Build history of the part. All positions in model axes, mm. Face numbers are marked on the shaded views. A direction names the side the tool comes from. Coordinates: 2 decimals unless noted, no trailing zeros. Order: outer loops, then holes, each group sorted by start corner. A loop starts at its lowest first (then second) coordinate and runs counter-clockwise, first axis right, second up. Notation, with made-up numbers: M -12,78.25 L 14,78.25 A18 ccw 14,102.25 Z; hole C 43,69 d4. An arc over 180 degrees is marked long. Write item = value, one per line. Start each with the question number.
Q1. Band-saw the part on A-A on x = 14.75. Write the cut outline in (y, z), plus the area to 3 significant figures.
Q2. Pull direction X, two halves, no side cores. Call the marked faces 1, 2 and 3: released by +X, released by -X, zero draft, split by the parting line, or undercut.
Q3. 3-axis set-ups, long thin cutter, end or side, ignore diameter. For the marked faces 4 and 5: which of +Z, -Z, +X, -X, +Y, -Y reach the whole face in a straight line?
Q4. Band-saw the part on D-D on y = -5.5. Write the cut outline in (x, z).
Q5. Band-saw the part on C-C on y = -7.5. Write the cut outline in (x, z).
Q6. Pin check, flat tips, straight feed: P1, Ø7, axis at x = 12.5, y = 1, coming from the -Z side; P2, Ø1.5, axis at y = -0.5, z = -13.5, coming from the +X side. Stop position of each tip, or through.
Q7. Drill centre lines: probe 1 along Y at (x, z) = (8, -4.75); probe 2 along Z at (x, y) = (10.5, -5.75); probe 3 along X at (y, z) = (-3.75, -11). Where is each one in solid material? Low to high.
Q8. Band-saw the part on B-B on z = -11.25. Write the cut outline in (x, y).
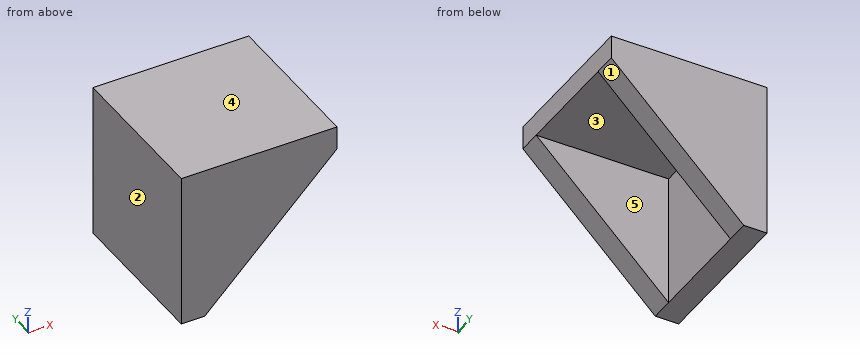
```python
from build123d import *

# Parameters (mm, degrees)
EXTRUDE_1_DEPTH = 10
EXTRUDE_START   = -10
EXTRUDE_2_DEPTH = 3


with BuildPart() as part:
    # Sketch 1 → Extrude 1 (new, symmetric)
    with BuildSketch(Plane(origin=(0, 0, 0), x_dir=(1, 0, 0), z_dir=(0, 1, 0))):
        Polygon((20, 0), (0, 0), (0, 20), (3, 20), (3, 3), (20, 3), align=None)
    extrude(amount=EXTRUDE_1_DEPTH, both=True)

    # Sketch 1_3 → Extrude 2 (add)
    with BuildSketch(Plane(origin=(0, 0, 0), x_dir=(1, 0, 0), z_dir=(0, 1, 0)).offset(EXTRUDE_START)):
        Polygon((3, 20), (20, 3), (3, 3), align=None)
    extrude_2 = extrude(amount=EXTRUDE_2_DEPTH)

    # Mirror 2: Extrude 2 across plane
    add(extrude_2.mirror(Plane.ZX))


solid = part.part
```
Recorded:
q1.outline = M -10,-8.25 L -7,-8.25 L -7,-3 L 7,-3 L 7,-8.25 L 10,-8.25 L 10,0 L -10,0 Z
q1.area = 91.5 mm2
q2.face_1 = released by +X
q2.face_2 = released by -X
q2.face_3 = zero draft
q3.face_4 = +Z, +X, -X, +Y, -Y
q3.face_5 = -Z, +X
q4.outline = M 0,-20 L 3,-20 L 3,-3 L 20,-3 L 20,0 L 0,0 Z
q5.outline = M 0,-20 L 3,-20 L 20,-3 L 20,0 L 0,0 Z
q6.P1 = -3
q6.P2 = 3
q7.probe_1 = -10 to -7, 7 to 10
q7.probe_2 = -3 to 0
q7.probe_3 = 0 to 3
q8.outline = M 0,-10 L 11.75,-10 L 11.75,-7 L 3,-7 L 3,7 L 11.75,7 L 11.75,10 L 0,10 Z
